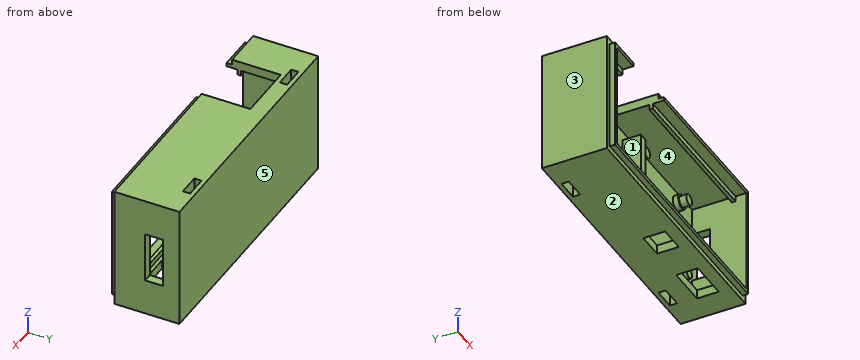
from build123d import *

# Parameters (mm, degrees)
SKETCH1_W             = 73
SKETCH1_H             = 34
BASE_DEPTH            = 4.5
SKETCH21_W            = 73
SKETCH21_H            = 34
EXTRUDE_UP_DEPTH      = 13.5
SKETCH22_W            = 68
SKETCH22_H            = 29
CUT_DOWN_DEPTH        = 13.5
SKETCH27_R            = 2
BOSS_EXTRUDE15_DEPTH  = 1.5
SKETCH29_R            = 2
BOSS_EXTRUDE16_DEPTH  = 1.5
SKETCH30_R            = 2
BOSS_EXTRUDE17_DEPTH  = 1.5
SKETCH28_R            = 2
BOSS_EXTRUDE18_DEPTH  = 1.5
SKETCH31_R            = 1.5
BOSS_EXTRUDE19_DEPTH  = 2
SKETCH32_R            = 1.5
BOSS_EXTRUDE20_DEPTH  = 2
SKETCH33_R            = 1.5
BOSS_EXTRUDE21_DEPTH  = 2
SKETCH34_R            = 1.5
BOSS_EXTRUDE22_DEPTH  = 2
SKETCH39_W            = 19
SKETCH39_H            = 1.3
WALL_SLIT_DEPTH       = 1.5
SKETCH41_W            = 2.5
SKETCH41_H            = 24
OUTSIDE_BLOCK_DEPTH   = 5
SKETCH44_W            = 2.5
SKETCH44_H            = 24
INSIDE_BLOCK_DEPTH    = 5
SKETCH62_W            = 70
SKETCH62_H            = 31
RAISE_LIP_DEPTH       = 1.5
SKETCH74_W            = 16
SKETCH74_H            = 15
USB_HOLE_DEPTH        = 2.5
SKETCH63_W            = 68
SKETCH63_H            = 29
CUT_LIP_DEPTH         = 1.5
SKETCH47_W            = 6
SKETCH47_H            = 2
TOP_TIE_HOLE_DEPTH    = 34
SKETCH48_W            = 6
SKETCH48_H            = 2
BOTTOM_TIE_HOLE_DEPTH = 34
SKETCH56_W            = 14
SKETCH56_H            = 5
WIRE_HOLE_DEPTH       = 2.5
SKETCH68_W            = 68
SKETCH68_H            = 1
RIGHT_LEDGE_DEPTH     = 1.5
SKETCH67_W            = 43.4
SKETCH67_H            = 1
SKETCH67_W_2          = 8.6
LEFT_LEDGE_DEPTH      = 1.5
SKETCH69_W            = 11
SKETCH69_H            = 6
SWITCH_HOLE_DEPTH     = 2.5
SKETCH70_W            = 7.245173121
SKETCH70_H            = 6
POWER_HOLE_DEPTH      = 2.5


with BuildPart() as part:
    # Sketch1 → base (new body)
    with BuildSketch(Plane(origin=(0, 0, 0), x_dir=(1, 0, 0), z_dir=(0, 1, 0))):
        with Locations((5.291578947, 0.823157895)):
            Rectangle(SKETCH1_W, SKETCH1_H)
    extrude(amount=BASE_DEPTH)

    # Sketch21 → extrude up (add)
    with BuildSketch(Plane(origin=(0, 0, 0), x_dir=(-1, 0, 0), z_dir=(0, -1, 0))):
        with Locations((-5.291578947, 0.823157895)):
            Rectangle(SKETCH21_W, SKETCH21_H)
    extrude(amount=EXTRUDE_UP_DEPTH)

    # Sketch22 → cut down (cut)
    with BuildSketch(Plane(origin=(0, -13.5, 0), x_dir=(-1, 0, 0), z_dir=(0, -1, 0))):
        with Locations((-5.291578947, 0.823157895)):
            Rectangle(SKETCH22_W, SKETCH22_H)
    extrude(amount=-CUT_DOWN_DEPTH, mode=Mode.SUBTRACT)

    # Sketch27 → Boss-Extrude15 (add)
    with BuildSketch(Plane.XZ):
        with Locations(Location((31.141578947, -11.923157895, 0), (0, 0, 270))):
            Circle(SKETCH27_R)
    extrude(amount=BOSS_EXTRUDE15_DEPTH)

    # Sketch29 → Boss-Extrude16 (add)
    with BuildSketch(Plane.XZ):
        with Locations(Location((9.041578947, -11.923157895, 0), (0, 0, 270))):
            Circle(SKETCH29_R)
    extrude(amount=BOSS_EXTRUDE16_DEPTH)

    # Sketch30 → Boss-Extrude17 (add)
    with BuildSketch(Plane.XZ):
        with Locations(Location((9.041578947, 10.276842105, 0), (0, 0, 270))):
            Circle(SKETCH30_R)
    extrude(amount=BOSS_EXTRUDE17_DEPTH)

    # Sketch28 → Boss-Extrude18 (add)
    with BuildSketch(Plane.XZ):
        with Locations(Location((31.141578947, 10.276842105, 0), (0, 0, 270))):
            Circle(SKETCH28_R)
    extrude(amount=BOSS_EXTRUDE18_DEPTH)

    # Sketch31 → Boss-Extrude19 (add)
    with BuildSketch(Plane.XZ.offset(1.5)):
        with Locations(Location((31.141578947, -11.923157895, 0), (0, 0, 270))):
            Circle(SKETCH31_R)
    extrude(amount=BOSS_EXTRUDE19_DEPTH)

    # Sketch32 → Boss-Extrude20 (add)
    with BuildSketch(Plane.XZ.offset(1.5)):
        with Locations(Location((9.041578947, -11.923157895, 0), (0, 0, 270))):
            Circle(SKETCH32_R)
    extrude(amount=BOSS_EXTRUDE20_DEPTH)

    # Sketch33 → Boss-Extrude21 (add)
    with BuildSketch(Plane.XZ.offset(1.5)):
        with Locations(Location((9.041578947, 10.276842105, 0), (0, 0, 270))):
            Circle(SKETCH33_R)
    extrude(amount=BOSS_EXTRUDE21_DEPTH)

    # Sketch34 → Boss-Extrude22 (add)
    with BuildSketch(Plane.XZ.offset(1.5)):
        with Locations(Location((31.141578947, 10.276842105, 0), (0, 0, 270))):
            Circle(SKETCH34_R)
    extrude(amount=BOSS_EXTRUDE22_DEPTH)

    # Sketch39 → wall slit (cut)
    with BuildSketch(Plane.XY.offset(-15.323157895)):
        with Locations((-11.708421053, -4.85)):
            Rectangle(SKETCH39_W, SKETCH39_H)
    extrude(amount=-WALL_SLIT_DEPTH, mode=Mode.SUBTRACT)

    # Sketch41 → outside block (add)
    with BuildSketch(Plane.XZ):
        with Locations((-27.458421053, -0.823157895)):
            Rectangle(SKETCH41_W, SKETCH41_H)
    extrude(amount=OUTSIDE_BLOCK_DEPTH)

    # Sketch44 → inside block (add)
    with BuildSketch(Plane.XZ):
        with Locations((4.041578947, -0.823157895)):
            Rectangle(SKETCH44_W, SKETCH44_H)
    extrude(amount=INSIDE_BLOCK_DEPTH)

    # Sketch62 → raise lip (add)
    with BuildSketch(Plane.XZ.offset(13.5)):
        with Locations((5.291578947, -0.823157895)):
            Rectangle(SKETCH62_W, SKETCH62_H)
    extrude(amount=RAISE_LIP_DEPTH)

    # Sketch74 → usb hole (cut)
    with BuildSketch(Plane(origin=(0, 0, 13.676842105), x_dir=(-1, 0, 0), z_dir=(0, 0, -1))):
        with Locations((12.108421053, -7.5)):
            Rectangle(SKETCH74_W, SKETCH74_H)
    extrude(amount=-USB_HOLE_DEPTH, mode=Mode.SUBTRACT)

    # Sketch63 → cut lip (cut)
    with BuildSketch(Plane.XZ.offset(15)):
        with Locations((5.291578947, -0.823157895)):
            Rectangle(SKETCH63_W, SKETCH63_H)
    extrude(amount=-CUT_LIP_DEPTH, mode=Mode.SUBTRACT)

    # Sketch47 → top tie hole (cut)
    with BuildSketch(Plane.XY.offset(16.176842105)):
        with Locations((30.791578947, 2.25)):
            Rectangle(SKETCH47_W, SKETCH47_H)
    extrude(amount=-TOP_TIE_HOLE_DEPTH, mode=Mode.SUBTRACT)

    # Sketch48 → bottom tie hole (cut)
    with BuildSketch(Plane.XY.offset(16.176842105)):
        with Locations((-20.208421053, 2.25)):
            Rectangle(SKETCH48_W, SKETCH48_H)
    extrude(amount=-BOTTOM_TIE_HOLE_DEPTH, mode=Mode.SUBTRACT)

    # Sketch56 → wire hole (cut)
    with BuildSketch(Plane.ZY.offset(-39.291578947)):
        with Locations((-0.823157895, -2.5)):
            Rectangle(SKETCH56_W, SKETCH56_H)
    extrude(amount=-WIRE_HOLE_DEPTH, mode=Mode.SUBTRACT)

    # Sketch68 → right ledge (add)
    with BuildSketch(Plane.XY.offset(-15.323157895)):
        with Locations((5.291578947, -11.5)):
            Rectangle(SKETCH68_W, SKETCH68_H)
    extrude(amount=RIGHT_LEDGE_DEPTH)

    # Sketch67 → left ledge (add)
    with BuildSketch(Plane(origin=(0, 0, 13.676842105), x_dir=(-1, 0, 0), z_dir=(0, 0, -1))):
        with Locations((-17.591578947, -11.5)):
            Rectangle(SKETCH67_W, SKETCH67_H)
        with Locations((24.408421053, -11.5)):
            Rectangle(SKETCH67_W_2, SKETCH67_H)
    extrude(amount=LEFT_LEDGE_DEPTH)

    # Sketch69 → switch hole (cut)
    with BuildSketch(Plane.XY.offset(-15.323157895)):
        with Locations((28.791578947, -7)):
            Rectangle(SKETCH69_W, SKETCH69_H)
    extrude(amount=-SWITCH_HOLE_DEPTH, mode=Mode.SUBTRACT)

    # Sketch70 → power hole (cut)
    with BuildSketch(Plane(origin=(0, 0, -17.823157895), x_dir=(-1, 0, 0), z_dir=(0, 0, -1))):
        with Locations((-9.668992387, -7)):
            Rectangle(SKETCH70_W, SKETCH70_H)
    extrude(amount=-POWER_HOLE_DEPTH, mode=Mode.SUBTRACT)


solid = part.part
CAD build for the part. Positions are in the model's coordinates, mm. Face numbers are marked on the shaded views. A direction names the side the tool comes from. Give positions to 0.01 mm unless a question says otherwise; leave off trailing zeros. Write each loop counter-clockwise with the first axis right and the second up, starting at its lowest first coordinate (ties: lowest second). Pieces come first, ordered by that corner, then holes. Notation, with made-up numbers: (37.25, 51) -> (58.25, 51) arc R17 cw to (58.25, 79) -> close; hole circle Ø9 at (58.25, 79). An arc over 180 degrees is marked (long way). Return JSON: item names as keys, results as strings.
Item 1: Band-saw the part on D-D (x = -10). List the corners of the cut face in (y, z).
Answer below:
{"outline": "(-15, -16.32) -> (-13.5, -16.32) -> (-13.5, -17.82) -> (4.5, -17.82) -> (4.5, 16.18) -> (0, 16.18) -> (0, -15.32) -> (-4.2, -15.32) -> (-4.2, -16.82) -> (-5.5, -16.82) -> (-5.5, -15.32) -> (-11, -15.32) -> (-11, -13.82) -> (-12, -13.82) -> (-12, -15.32) -> (-15, -15.32) -> close"}
Item 2: Tool access for the marked faces 1 and 2: list every direction of +Z, -Z, +X, -X, +Y, -Y with a clear straight run to the whole face (end or side of a thin tool).
Answer below:
{"face 1": "-Y", "face 2": "-Z, +X, -X, +Y, -Y"}
Item 3: Band-saw the part on C-C (y = -7.5). List the corners of the cut face in (x, z), then the cut area to 3 significant figures.
Answer below:
{"outline": "(-31.21, -17.82) -> (6.05, -17.82) -> (6.05, -15.32) -> (-28.71, -15.32) -> (-28.71, 13.68) -> (-20.11, 13.68) -> (-20.11, 16.18) -> (-31.21, 16.18) -> close; (-4.11, 13.68) -> (39.29, 13.68) -> (39.29, -15.32) -> (34.29, -15.32) -> (34.29, -17.82) -> (41.79, -17.82) -> (41.79, 16.18) -> (-4.11, 16.18) -> close; (13.29, -17.82) -> (23.29, -17.82) -> (23.29, -15.32) -> (13.29, -15.32) -> close", "area": "424 mm2"}
Item 4: Drop flat-ended pins along their axis: pin 1 (17 mm diameter, centred on x = 10, z = 0, fed in from -Y); pin 2 (1.6 mm diameter, centred on x = -23, z = 12.5, fed in from -Y); pin 3 (0.8 mm diameter, centred on x = 17, y = -14, fed in from -Z). Give the stop position or say it passes through.
Answer below:
{"pin 1": "stops at y = -5", "pin 2": "stops at y = -12", "pin 3": "stops at z = -16.32"}
Item 5: Drill centre lines: probe 1 along Z at (x, y) = (5, -4.5); probe 2 along X at (y, z) = (-6.75, 0); probe 3 along X at (y, z) = (-1, 0). Where is each one in solid material? Low to high.
Answer below:
{"probe 1": "z = -17.82 to -15.32, -12.82 to 11.18, 13.68 to 16.18", "probe 2": "x = -31.21 to -28.71, 39.29 to 41.79", "probe 3": "x = -31.21 to -26.21, 2.79 to 5.29"}
Item 6: Two-plate mould, pull along Y, no slides. Class the marked faces 3, 4 and 5: +Y half, -Y half, draft (parallel to the pull), parting line (faces both ways), or undercut.
Answer below:
{"face 3": "draft", "face 4": "undercut", "face 5": "+Y half"}
Item 7: Band-saw the part on B-B (x = -18.5). List the corners of the cut face in (y, z), then the cut area to 3 significant figures.
Answer below:
{"outline": "(-15, -16.32) -> (-13.5, -16.32) -> (-13.5, -17.82) -> (1.25, -17.82) -> (1.25, 16.18) -> (0, 16.18) -> (0, -15.32) -> (-4.2, -15.32) -> (-4.2, -16.82) -> (-5.5, -16.82) -> (-5.5, -15.32) -> (-11, -15.32) -> (-11, -13.82) -> (-12, -13.82) -> (-12, -15.32) -> (-15, -15.32) -> close; (3.25, -17.82) -> (4.5, -17.82) -> (4.5, 16.18) -> (3.25, 16.18) -> close", "area": "120 mm2"}
Item 8: Band-saw the part on A-A (z = -1.5). List the corners of the cut face in (x, y).
Answer below:
{"outline": "(-31.21, -13.5) -> (-29.71, -13.5) -> (-29.71, -15) -> (-28.71, -15) -> (-28.71, -5) -> (-26.21, -5) -> (-26.21, 0) -> (2.79, 0) -> (2.79, -5) -> (5.29, -5) -> (5.29, 0) -> (41.79, 0) -> (41.79, 4.5) -> (-31.21, 4.5) -> close; (39.29, -15) -> (40.29, -15) -> (40.29, -13.5) -> (41.79, -13.5) -> (41.79, -5) -> (39.29, -5) -> close; hole (-23.21, 1.25) -> (-17.21, 1.25) -> (-17.21, 3.25) -> (-23.21, 3.25) -> close; hole (27.79, 1.25) -> (33.79, 1.25) -> (33.79, 3.25) -> (27.79, 3.25) -> close"}
